Autodesk Inventor part; units mm, degrees
ref_plane "YZ Plane" through (0, 0, 0) normal (1, 0, 0) x (0, 1, 0)
ref_plane "XZ Plane" through (0, 0, 0) normal (0, 1, 0) x (-1, 0, 0)
ref_plane "XY Plane" through (0, 0, 0) normal (0, 0, 1) x (1, 0, 0)
sketch "Эскиз3" plane through (0, 0, 0) normal (0, 0, 1) x (1, 0, 0)
  line L0 (-20.1552, 0) -> (30.6288, 0)
  line L1 (15, 15) -> (12, 15)
  line L2 (15, 5) -> (15, 15)
  line L3 (-4, 3.175) -> (-15, 3.175)
  line L4 (-15, 3.175) -> (-15, 15)
  line L5 (4, 5) -> (15, 5)
  line L6 (-30.312, 0) -> (40.7856, 0)
  line L7 (4, 5) -> (0, 5)
  line L8 (0, 5) -> (0, 3.175)
  line L9 (0, 3.175) -> (-4, 3.175)
  line L10 (12, 15) -> (-15, 15)
  dimension "d43" = 6.35
  dimension "d50" = 30
  dimension "d51" = 10
  dimension "d61" = 30
revolve "Вращение5" add sketch "Эскиз3" angle 360 about axis through (-20.1552, 0, 0) along (1, 0, 0)
properties part number "DR-30-6,35x10"
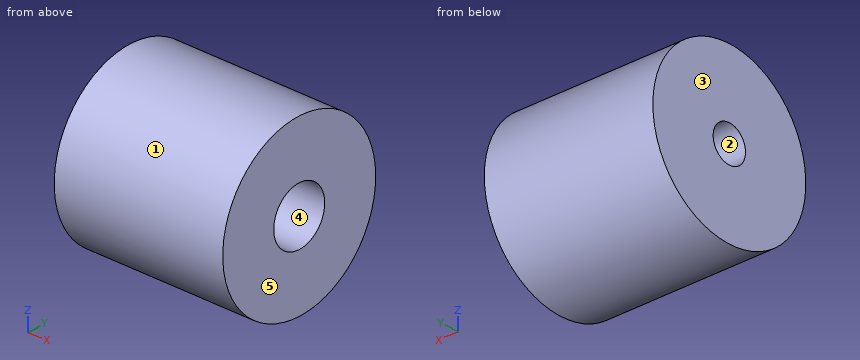
Build history of the part. All positions in model axes, mm. Face numbers are marked on the shaded views. A direction names the side the tool comes from. Round coordinates to 2 decimals unless told otherwise and drop trailing zeros. Write each loop counter-clockwise with the first axis right and the second up, starting at its lowest first coordinate (ties: lowest second). Pieces come first, ordered by that corner, then holes.
1) 3-axis set-ups, long thin cutter, end or side, ignore diameter. For the marked faces 4 and 5: which of +Z, -Z, +X, -X, +Y, -Y reach the whole face in a straight line?
2) Drill centre lines: probe 1 along Z at (x, y) = (5.5, 0); probe 2 along Z at (x, y) = (-5, 0) (3 decimals); probe 3 along Y at (x, z) = (8.5, -0.25). Where is each one in solid material? Low to high.
3) Band-saw the part on C-C, the plane x = -2.25. List the corners of the cut face in (y, z) (3 decimals).
4) Band-saw the part on A-A, the plane z = 0. List the corners of the cut face in (x, y) (3 decimals), and give its area (3 significant figures).
5) Pin check, flat tips, straight feed: pin 1 (6 mm diameter, centred on x = 2, z = 11.5, fed in from +Y); pin 2 (5 mm diameter, centred on x = 5, y = 5.5, fed in from -Z); pin 3 (11 mm diameter, centred on y = 0, z = -1.5, fed in from +X); pin 4 (5.5 mm diameter, centred on y = 0, z = 0, fed in from -X). Stop position of each tip, or through.
6) Mould opens along Y. For the marked faces 1, 2 and 3 say: +Y half, -Y half, draft (parallel to the pull), parting line (faces both ways), or undercut.
7) Band-saw the part on D-D, the plane y = -4. List the corners of the cut face in (x, z), and give its area (3 significant figures).
Ans:
1. face 4: +X
1. face 5: +Z, -Z, +X, +Y, -Y
2. probe 1: z = -15 to -5, 5 to 15
2. probe 2: z = -15 to -3.175, 3.175 to 15
2. probe 3: y = -15 to -4.99, 4.99 to 15
3. outline: circle Ø30 at (0, 0); hole circle Ø6.35 at (0, 0)
4. outline: (-15, -15) - (15, -15) - (15, -5) - (0, -5) - (0, -3.175) - (-15, -3.175) - close; (-15, 3.175) - (0, 3.175) - (0, 5) - (15, 5) - (15, 15) - (-15, 15) - close
4. area: 655 mm2
5. pin 1: stops at y = 12.36
5. pin 2: stops at z = -14.7
5. pin 3: stops at x = 15
5. pin 4: passes through
6. face 1: parting line
6. face 2: undercut
6. face 3: draft
7. outline: (-15, -14.46) - (15, -14.46) - (15, -3) - (0, -3) - (0, 3) - (15, 3) - (15, 14.46) - (-15, 14.46) - close
7. area: 777 mm2
